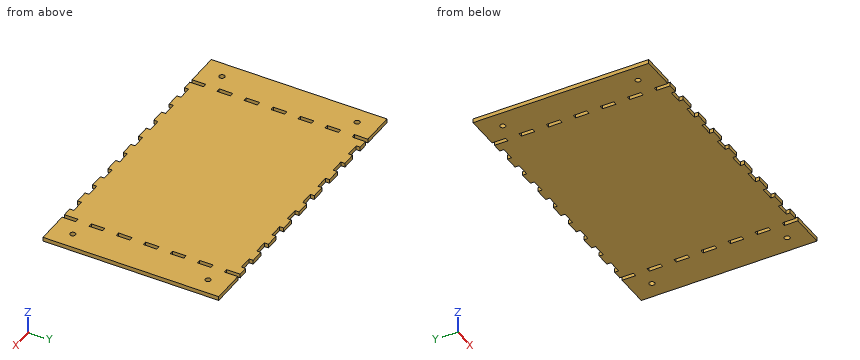
```python
from build123d import *

# Parameters (mm, degrees)
F0_W     = 220
F0_H     = 130
F1_DEPTH = 3
F2_W     = 10
F2_H     = 3
F2_W_2   = 3
F2_H_2   = 10
F3_DEPTH = 3.001
F4_R     = 2
F5_DEPTH = 3.001


with BuildPart() as f1:
    # F0 (on Top) → F1 (new body)
    with BuildSketch(Plane.XY):
        Rectangle(F0_W, F0_H)
    extrude(amount=F1_DEPTH)

    # F2 (on face) → F3 (cut, through all)
    with BuildSketch(Plane.XY.offset(3)):
        with Locations((-70, -63.5)):
            Rectangle(F2_W, F2_H)
        with Locations((-50, -63.5)):
            Rectangle(F2_W, F2_H)
        with Locations((-30, -63.5)):
            Rectangle(F2_W, F2_H)
        with Locations((-10, -63.5)):
            Rectangle(F2_W, F2_H)
        with Locations((10, -63.5)):
            Rectangle(F2_W, F2_H)
        with Locations((30, -63.5)):
            Rectangle(F2_W, F2_H)
        with Locations((50, -63.5)):
            Rectangle(F2_W, F2_H)
        with Locations((70, -63.5)):
            Rectangle(F2_W, F2_H)
        with Locations((-83.5, -60)):
            Rectangle(F2_W_2, F2_H_2)
        with Locations((-83.5, -40)):
            Rectangle(F2_W_2, F2_H_2)
        with Locations((-83.5, -20)):
            Rectangle(F2_W_2, F2_H_2)
        with Locations((-83.5, 0)):
            Rectangle(F2_W_2, F2_H_2)
        with Locations((-83.5, 20)):
            Rectangle(F2_W_2, F2_H_2)
        with Locations((-83.5, 40)):
            Rectangle(F2_W_2, F2_H_2)
        with Locations((-83.5, 60)):
            Rectangle(F2_W_2, F2_H_2)
        with Locations((-50, 63.5)):
            Rectangle(F2_W, F2_H)
        with Locations((30, 63.5)):
            Rectangle(F2_W, F2_H)
        with Locations((-70, 63.5)):
            Rectangle(F2_W, F2_H)
        with Locations((70, 63.5)):
            Rectangle(F2_W, F2_H)
        with Locations((-10, 63.5)):
            Rectangle(F2_W, F2_H)
        with Locations((-30, 63.5)):
            Rectangle(F2_W, F2_H)
        with Locations((50, 63.5)):
            Rectangle(F2_W, F2_H)
        with Locations((10, 63.5)):
            Rectangle(F2_W, F2_H)
        with Locations((83.5, -40)):
            Rectangle(F2_W_2, F2_H_2)
        with Locations((83.5, -20)):
            Rectangle(F2_W_2, F2_H_2)
        with Locations((83.5, 40)):
            Rectangle(F2_W_2, F2_H_2)
        with Locations((83.5, 60)):
            Rectangle(F2_W_2, F2_H_2)
        with Locations((83.5, 20)):
            Rectangle(F2_W_2, F2_H_2)
        with Locations((83.5, -60)):
            Rectangle(F2_W_2, F2_H_2)
        with Locations((83.5, 0)):
            Rectangle(F2_W_2, F2_H_2)
    extrude(amount=-F3_DEPTH, mode=Mode.SUBTRACT)

    # F4 (on face) → F5 (cut, through all)
    with BuildSketch(Plane.XY.offset(3)):
        with Locations((97.5, 50)):
            Circle(F4_R)
        with Locations((97.5, -50)):
            Circle(F4_R)
        with Locations((-97.5, 50)):
            Circle(F4_R)
        with Locations((-97.5, -50)):
            Circle(F4_R)
    extrude(amount=-F5_DEPTH, mode=Mode.SUBTRACT)


solid = f1.part
```
Check sheet for the modelled part. Datum: model origin and axes. Units: mm. Give positions to 0.01 mm unless a question says otherwise; leave off trailing zeros. Use CSV: the item, a comma, the result in double quotes. Start each with the question number.
Q1. Cross-section at A-A on z = 2.45. Count the separate pieces of the cut face and the enclosed holes in it, and give its area (3 significant figures).
Q2. Scan lines: line 1 along Y through (x, z) = (-97.5, 1.45); line 2 along X through (y, z) = (-40.5, 2.65); line 3 along Y through (x, z) = (-73, 0.4). Record each from-to range of solid material in increasing order.
Q3. Depth check by flat-ended pin: P1, Ø0.9, axis at x = 9, z = 1, coming from the -Y side; P2, Ø0.9, axis at x = -49.5, z = 2, coming from the +Y side; P3, Ø1.5, axis at x = -83, z = 2, coming from the -Y side. Enter the tip coordinate at first touch or a pass-through.
Working result:
1,separate pieces,"1"
1,enclosed holes,"14"
1,area,"27,600 mm^2"
2,line 1,"y = -65 to -52, -48 to 48, 52 to 65"
2,line 2,"x = -110 to -85, -82 to 82, 85 to 110"
2,line 3,"y = -62 to 62"
3,P1,"stops at y = -62"
3,P2,"stops at y = 62"
3,P3,"stops at y = -55"
